Verification items for the finished model (mm, model axes). Face numbers are marked on the shaded views. A direction names the side the tool comes from. Coordinates: 2 decimals unless noted, no trailing zeros. Write each loop counter-clockwise with the first axis right and the second up, starting at its lowest first coordinate (ties: lowest second). Pieces come first, ordered by that corner, then holes. Notation, with made-up numbers: M 59.5,-29.5 L 89.5,-29.5 A28 cw 89.5,4.5 Z; hole C 63.25,-26.5 d9. An arc over 180 degrees is marked long. One line per item, written item: value.
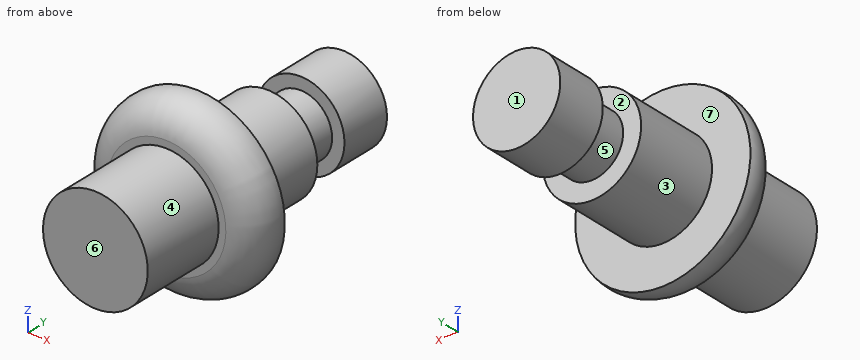
Autodesk Inventor part; units mm, degrees
ref_plane "YZ Plane" through (0, 0, 0) normal (1, 0, 0) x (0, 1, 0)
ref_plane "XZ Plane" through (0, 0, 0) normal (0, 1, 0) x (-1, 0, 0)
ref_plane "XY Plane" through (0, 0, 0) normal (0, 0, 1) x (1, 0, 0)
sketch "Sketch1" plane through (0, 0, 0) normal (0, 1, 0) x (-1, 0, 0)
  circle A0 centre (0, 0) radius 3.6
  dimension "d0" = 7.2
extrude "Extrusion1" add sketch "Sketch1" along normal blind 6
sketch "Sketch2" plane through (0, 0, 0) normal (1, 0, 0) x (0, 1, 0)
  line L0 (6, -3.6) -> (6, 3.6)
  line L1 (6, 0) -> (8.6201, 0)
  line L2 (8.6201, 0) -> (8.6201, -6.024)
  line L3 (6, -3.6) -> (6, -4.0964)
  arc A0 (6, -4.0964) -> (8.6201, -6.024) centre (8.1594, -3.9057) ccw
  point P0 (0, 0)
revolve "Revolution1" add sketch "Sketch2" angle 360 about axis through (0, 6, 0) along (0, 1, 0)
sketch "Sketch3" plane through (0, 8.6201, 0) normal (0, 1, 0) x (1, 0, 0)
  circle A0 centre (0, 0) radius 3.385
  dimension "d4" = 6.77
extrude "Extrusion2" add sketch "Sketch3" along normal blind 6
sketch "Sketch4" plane through (0, 14.6201, 0) normal (0, 1, 0) x (1, 0, 0)
  circle A0 centre (0, 0) radius 2.15
  dimension "d7" = 4.3
extrude "Extrusion3" add sketch "Sketch4" along normal blind 2.77
sketch "Sketch5" plane through (0, 17.3901, 0) normal (0, 1, 0) x (1, 0, 0)
  circle A0 centre (0, 0) radius 3
  dimension "d10" = 6
extrude "Extrusion4" add sketch "Sketch5" along normal blind 3.6
thread "Thread1"
properties part number "BLACKBUTTON"
Item 1: Draft check along Y on the marked faces 4, 5, 6 and 7. Enter one of: released by +Y, released by -Y, zero draft, split by the parting line, or undercut.
The answers:
face 4: zero draft
face 5: undercut
face 6: released by -Y
face 7: released by +Y
Item 2: Scan lines: line 1 (Y direction, x = 2.75, z = 0.5); line 2 (Y direction, x = -3, z = 1.25); line 3 (Y direction, x = 1.5, z = 3.5). Record each from-to range of solid material in increasing order.
The answers:
line 1: y = 0 to 14.62, 17.39 to 20.99
line 2: y = 0 to 14.62
line 3: y = 6 to 8.62
Item 3: Cross-section at B-B, the plane y = 3.25. Enter the section's corners in (x, z).
The answers:
outline: C 0,0 d7.2
Item 4: Cross-section at A-A, the plane x = 0. Enter the section's corners in (y, z) (3 decimals), and give its area (3 significant figures).
The answers:
outline: M 0,-3.6 L 6,-3.6 L 6,-4.096 A2.168 ccw 8.62,-6.024 L 8.62,-3.385 L 14.62,-3.385 L 14.62,-2.15 L 17.39,-2.15 L 17.39,-3 L 20.99,-3 L 20.99,3 L 17.39,3 L 17.39,2.15 L 14.62,2.15 L 14.62,3.385 L 8.62,3.385 L 8.62,6.024 A2.168 ccw 6,4.096 L 6,3.6 L 0,3.6 Z
area: 147 mm²
Item 5: Access from +Z, -Z, +X, -X, +Y, -Y to the whole of each face (thin tool, end or side, straight path). Record for the marked faces 1, 2 and 3.
The answers:
face 1: +Z, -Z, +X, -X, +Y
face 2: none
face 3: +Y
Item 6: Cross-section at C-C, the plane y = 6.5. Enter the section's corners in (x, z).
The answers:
outline: C 0,0 d10.6
Item 7: Go/stop test with flat-tipped pins: P1, Ø6, axis at y = 6, z = -1.5, coming from the +X side; P2, Ø6, axis at y = 12.5, z = 0, coming from the +X side (3 decimals); P3, Ø3, axis at y = 3.5, z = -3.5, coming from the -X side; P4, Ø1, axis at x = -0.5, z = -4.5, coming from the -Y side. Record where each tip stops, or that it passes through.
The answers:
P1: stops at x = 6.07
P2: stops at x = 3.385
P3: stops at x = -2.99
P4: stops at y = 6
